Autodesk Inventor part; units mm, degrees
ref_plane "YZ Plane" through (0, 0, 0) normal (1, 0, 0) x (0, 1, 0)
ref_plane "XZ Plane" through (0, 0, 0) normal (0, 1, 0) x (-1, 0, 0)
ref_plane "XY Plane" through (0, 0, 0) normal (0, 0, 1) x (1, 0, 0)
sketch "Sketch9" plane through (0, 0, 0) normal (0, 0, 1) x (1, 0, 0)
  line L0 (44, 0) -> (44, -29)
  line L1 (0, -29) -> (0, 0)
  line L2 (44, 0) -> (38, 0)
  line L3 (0, -29) -> (6, -29)
  circle A0 centre (9, -32) radius 1.5
  circle A1 centre (35, -32) radius 1.5
  circle A2 centre (35, 3) radius 1.5
  circle A3 centre (9, 3) radius 1.5
  line L4 (0, 0) -> (0, 10)
  line L5 (0, 10) -> (-10, 10)
  line L6 (44, -29) -> (54, -29)
  line L7 (54, -29) -> (54, -39)
  line L8 (-10, 10) -> (54, 10)
  line L9 (54, 10) -> (54, -39)
  line L10 (54, -39) -> (-10, -39)
  line L11 (-10, -39) -> (-10, 10)
  line L12 (-10, 10) -> (-10, 13)
  line L13 (-10, 13) -> (-13, 13)
  line L14 (54, -39) -> (54, -42)
  line L15 (54, -42) -> (57, -42)
  line L16 (57, -42) -> (-13, -42)
  line L17 (-13, -42) -> (-13, 13)
  line L18 (-13, 13) -> (57, 13)
  line L19 (57, 13) -> (57, -42)
  circle A4 centre (9, 3) radius 3
  circle A5 centre (35, 3) radius 3
  circle A6 centre (35, -32) radius 3
  circle A7 centre (9, -32) radius 3
  dimension "d22" = 3
  dimension "d23" = 3
  dimension "d24" = 3
  dimension "d25" = 3
  dimension "d26" = 6
  dimension "d27" = 6
  dimension "d29" = 6
  dimension "d30" = 6
extrude "Extrusion1" add sketch "Sketch9" along normal blind 3 contours L8 L9 L7 L10 L11 L5 | L5 L12 L18 L19 L15 L14 L7 L9 L8 | L11 L10 L14 L16 L17 L13 L12
sketch "Sketch10" plane through (0, 0, 3) normal (0, 0, 1) x (1, 0, 0)
  line L0 (57, -42) -> (57, 13)
  line L1 (57, 11) -> (57, 10)
  line L2 (57, 13) -> (-13, 13)
  line L3 (55, 13) -> (54, 13)
  line L4 (54, 13) -> (54, 10)
  line L5 (57, 10) -> (57, 9)
  line L6 (54, 13) -> (53, 13)
  line L7 (53, 13) -> (53, 9)
  line L8 (-13, 13) -> (-13, -42)
  line L9 (-13, -40) -> (-13, -38)
  arc A0 (-13, -40) -> (-11, -42) centre (-11, -40) ccw
  line L10 (-11, -42) -> (-9, -42)
  line L11 (-13, -38) -> (-9, -38)
  line L12 (-9, -38) -> (-9, -42)
  line L13 (-9, -42) -> (-13, -42)
  line L14 (-13, -42) -> (-13, -38)
  line L15 (-9, -38) -> (53, -38)
  line L16 (53, -38) -> (53, 9)
  line L17 (53, 9) -> (-9, 9)
  line L18 (-9, 9) -> (-9, -38)
  line L19 (-13, -38) -> (-9, -38)
  line L20 (-9, -38) -> (-9, -42)
  line L21 (-9, -42) -> (-13, -42)
  line L22 (-13, -42) -> (-13, -38)
  line L23 (-9, 9) -> (53, 9)
  line L24 (53, 9) -> (53, -38)
  line L25 (53, -38) -> (-9, -38)
  line L26 (-9, -38) -> (-9, 9)
  line L27 (-13.4447, 13.4817) -> (58.1663, 13.4817)
  line L28 (58.1663, 13.4817) -> (58.1663, -42.7185)
  line L29 (58.1663, -42.7185) -> (-13.4447, -42.7185)
  line L30 (-13.4447, -42.7185) -> (-13.4447, 13.4817)
  line L31 (-9, 9) -> (53, 9)
  line L32 (53, 9) -> (53, -38)
  line L33 (53, -38) -> (-9, -38)
  line L34 (-9, -38) -> (-9, 9)
  line L35 (-14.6617, 14.1825) -> (60.6079, 14.1825)
  line L36 (60.6079, 14.1825) -> (60.6079, -44.8629)
  line L37 (60.6079, -44.8629) -> (-14.6617, -44.8629)
  line L38 (-14.6617, -44.8629) -> (-14.6617, 14.1825)
  point P0 (0, 0)
  point P1 (57, -40)
  point P2 (-11, 13)
  point P3 (-13, 11)
  point P4 (-13, -40)
  point P5 (-13, -40)
  dimension "d36" = 1
  dimension "d37" = 1
  dimension "d38" = 1
  dimension "d39" = 1
  dimension "d40" = 2
  dimension "d41" = 2
extrude "Extrusion4" cut sketch "Sketch10" against normal blind 6 contours L7 L17 L18 L11 L8 L2 | L11 L12 L10 A0 L8 | L27 L28 L29 L30
sketch "Sketch27" plane through (0, 0, 3) normal (0, 0, 1) x (1, 0, 0)
  point P0 (0, 0)
sketch "Sketch28" plane through (0, 0, 3) normal (0, 0, 1) x (1, 0, 0)
  line L0 (-9, 9) -> (53, 9)
  line L1 (53, 9) -> (53, -38)
  line L2 (53, -38) -> (-9, -38)
  line L3 (-9, -38) -> (-9, 9)
  point P0 (0, 0)
extrude "Extrusion7" add sketch "Sketch28" along normal blind 3
extrude "Extrusion8" cut sketch "Sketch9" against normal blind 6 contours A0 | A1 | A2 | A3
extrude "Extrusion9" cut sketch "Sketch9" along normal blind 82.9 contours A0 | A1 | A2 | A3
sketch "Sketch29" plane through (0, 0, 0) normal (0, 0, -1) x (-1, 0, 0)
  line L0 (17.5138, -45.6881) -> (10.4067, -45.6881)
  line L1 (10.4067, -45.6881) -> (10.4067, -38.0734)
  line L2 (10.4067, -38.0734) -> (17.5138, -38.0734)
  line L3 (17.5138, -38.0734) -> (17.5138, -45.6881)
  point P0 (0, 0)
extrude "Extrusion10" cut sketch "Sketch29" against normal blind 25.05
sketch "Sketch30" plane through (0, 0, 0) normal (0, 0, -1) x (-1, 0, 0)
  line L0 (-53, -38) -> (9, -38)
  line L1 (9, -38) -> (-53, -38)
  line L2 (-53, -38) -> (-53, 9.1187)
  line L3 (-53, 9.1187) -> (9, 9.1187)
  line L4 (9, 9.1187) -> (9, -38)
  point P0 (0, 0)
sketch "Sketch31" plane through (0, 0, 0) normal (0, 0, -1) x (-1, 0, 0)
  circle A0 centre (-9, -32) radius 3
  circle A1 centre (-9, -32) radius 4
  circle A2 centre (-35, -32) radius 1.5
  circle A3 centre (-9, 3) radius 3
  circle A4 centre (-9, 3) radius 4
  circle A5 centre (-35, 3) radius 3
  circle A6 centre (-35, 3) radius 4
  point P0 (0, 0)
extrude "Extrusion11" add sketch "Sketch30" along normal blind 2
extrude "Extrusion12" cut sketch "Sketch31" along normal blind 2 contours A0 | A3 | A5
sketch "Sketch32" plane through (0, 0, -2) normal (0, 0, -1) x (-1, 0, 0)
  point P0 (0, 0)
extrude "Extrusion14" cut sketch "Sketch31" along normal blind 8 contours A2
extrude "Extrusion15" cut sketch "Sketch9" against normal blind 4 contours A1 | A6
sketch "Sketch34" plane through (0, 0, -2) normal (0, 0, -1) x (-1, 0, 0)
  point P0 (0, 0)
sketch "Sketch35" plane through (0, 0, -2) normal (0, 0, -1) x (-1, 0, 0)
  line L0 (-53, -38) -> (-53, 9)
  line L1 (9, -38) -> (-53, -38)
  line L2 (-53, -38) -> (-53, 9)
  line L3 (-53, 9) -> (9, 9)
  line L4 (9, 9) -> (9, -38)
  line L5 (9, 9.1187) -> (-53, 9.1187)
  line L6 (9, 9) -> (-53, 9)
  line L7 (-53, 9) -> (-53, 9.1187)
  line L8 (-53, 9.1187) -> (9, 9.1187)
  line L9 (9, 9.1187) -> (9, 9)
  point P0 (0, 0)
extrude "Extrusion16" cut sketch "Sketch35" against normal blind 4 contours L7 L5 L9 L3
fillet "Fillet4" radius 2 4 edges at (-9, -38, 2) (53, -38, 2) (53, 9, 2) (-9, 9, 2)
properties part number "uchwyt_2"
Work out the finished part from the listing and answer in its coordinate system (mm). A direction names the side the tool comes from. Give positions to 0.01 mm unless a question says otherwise; leave off trailing zeros. Loops run counter-clockwise (first coordinate to the right, second up) from the corner with the lowest first, then second, coordinate; pieces in that order, holes last. Notation, with made-up numbers: (29.25, 8) -> (64.25, 8) arc R14 ccw to (64.25, 23) -> close; hole circle Ø11 at (40.25, -7.75). An arc over 180 degrees is marked (long way). One line per question, with ' | ' between items. Start each with the question number.
1) Section A-A, the plane z = 1.75 is taken. Determine the outline of the cut face in (x, y).
2) Each of these flat-tipped pins is pushed along its axis until it touches: pin 1 (5 mm diameter, centred on x = 9, y = -32, fed in from -Z); pin 2 (1.8 mm diameter, centred on x = 9, y = 3.5, fed in from -Z). Where does it stop, or does it pass through?
3) Straight lines are drawn through the part: L1, parallel to Y at x = 9, z = -0.5; L2, parallel to Y at x = 9, z = 4.9; L3, parallel to X at y = 3, z = 4.9. For each, find the intervals that lie inside material, in ascending order.
4) Determine the mould class of faces 3 (the face through (-8.4, -37.43, 1.94)), 4 (the face through (22, 9, 2)), 5 (the face through (10.3, 1.7, 3)) for opening direction Y: +Y half, -Y half, draft (parallel to the pull), parting line (faces both ways), or undercut.
5) Section B-B, the plane y = -32 is taken. Determine the outline of the cut face in (x, z), then the cut area to 3 significant figures.
6) Section C-C, the plane x = 35 is taken. Determine the outline of the cut face in (y, z), then the cut area to 3 significant figures.
7) For faces 1 (the face through (22, -14, 6)), 2 (the face through (36.3, -33.3, 3)), determine the directions among +Z, -Z, +X, -X, +Y, -Y from which every point of the face is accessible in a straight line to the end or side of a thin tool.
Resolved:
1) outline: (-9, -36) arc R2 ccw to (-7, -38) -> (51, -38) arc R2 ccw to (53, -36) -> (53, 7) arc R2 ccw to (51, 9) -> (-7, 9) arc R2 ccw to (-9, 7) -> close; hole circle Ø6 at (9, -32); hole circle Ø6 at (9, 3); hole circle Ø6 at (35, -32); hole circle Ø6 at (35, 3)
2) pin 1: z = 3 | pin 2: through
3) L1: -38 to -35, -29 to 0, 6 to 9 | L2: -38 to -33.5, -30.5 to 1.5, 4.5 to 9 | L3: -9 to 7.5, 10.5 to 33.5, 36.5 to 53
4) face 3: -Y half | face 4: +Y half | face 5: undercut
5) outline: (-9, -2) -> (6, -2) -> (6, 3) -> (7.5, 3) -> (7.5, 6) -> (-9, 6) -> close; (10.5, 3) -> (12, 3) -> (12, -2) -> (32, -2) -> (32, 3) -> (33.5, 3) -> (33.5, 6) -> (10.5, 6) -> close; (36.5, 3) -> (38, 3) -> (38, -2) -> (53, -2) -> (53, 6) -> (36.5, 6) -> close | area: 418 mm2
6) outline: (-38, -2) -> (-35, -2) -> (-35, 3) -> (-33.5, 3) -> (-33.5, 6) -> (-38, 6) -> close; (-30.5, 3) -> (-29, 3) -> (-29, -2) -> (0, -2) -> (0, 3) -> (1.5, 3) -> (1.5, 6) -> (-30.5, 6) -> close; (4.5, 3) -> (6, 3) -> (6, -2) -> (9, -2) -> (9, 6) -> (4.5, 6) -> close | area: 298 mm2
7) face 1: +Z, +X, -X, +Y, -Y | face 2: -Z
